from build123d import *

# Parameters (mm, degrees)
SKETCH1_W                       = 12.7
SKETCH1_H                       = 6.35
BOSS_EXTRUDE1_DEPTH             = 105.41
SKETCH2_W                       = 12.7
SKETCH2_H                       = 6.35
BOSS_EXTRUDE2_DEPTH             = 127
SKETCH3_W                       = 12.7
SKETCH3_H                       = 6.35
BOSS_EXTRUDE3_DEPTH             = 105.41
CUT_EXTRUDE1_DEPTH              = 128
LPATTERN1_COUNT                 = 5
LPATTERN1_PITCH                 = 19.05
F_9_64_0_14063_DIAMETER_HOLE1_D = 3.572002


with BuildPart() as part:
    # Sketch1 → Boss-Extrude1 (new body)
    with BuildSketch(Plane(origin=(0, 0, 0), x_dir=(1, 0, 0), z_dir=(0, 1, 0))):
        Rectangle(SKETCH1_W, SKETCH1_H)
    extrude(amount=-BOSS_EXTRUDE1_DEPTH)

    # Sketch2 → Boss-Extrude2 (add)
    with BuildSketch(Plane.XY.offset(3.175)):
        with Locations((0, -102.235)):
            Rectangle(SKETCH2_W, SKETCH2_H)
    extrude(amount=-BOSS_EXTRUDE2_DEPTH)

    # Sketch3 → Boss-Extrude3 (add)
    with BuildSketch(Plane.XZ.offset(105.41)):
        with Locations((0, -120.65)):
            Rectangle(SKETCH3_W, SKETCH3_H)
    extrude(amount=-BOSS_EXTRUDE3_DEPTH)

    # Sketch4 → Cut-Extrude1 (cut, through all)
    with BuildSketch(Plane(origin=(0, 0, -123.825), x_dir=(-1, 0, 0), z_dir=(0, 0, -1))):
        with BuildLine():
            Line((3.175, -10.16), (3.175, -17.78))
            ThreePointArc((3.175, -17.78), (0, -20.955), (-3.175, -17.78))
            Line((-3.175, -17.78), (-3.175, -10.16))
            ThreePointArc((-3.175, -10.16), (0, -6.985), (3.175, -10.16))
        make_face()
    cut_extrude1 = extrude(amount=-CUT_EXTRUDE1_DEPTH, mode=Mode.SUBTRACT)

    # LPattern1: Cut-Extrude1 ×5
    with Locations(*[(0, -i * LPATTERN1_PITCH, 0) for i in range(1, LPATTERN1_COUNT)]):
        add(cut_extrude1, mode=Mode.SUBTRACT)

    # 9/64 (0.14063) Diameter Hole1 (through all)
    with Locations(Plane(origin=(0, 0, -123.825), x_dir=(-1, 0, 0), z_dir=(0, 0, -1))):
        with Locations((0, -2.667)):
            Hole(F_9_64_0_14063_DIAMETER_HOLE1_D / 2)


solid = part.part
Geometry check sheet. Reference: the model listing, model coordinates, mm. A direction names the side the tool comes from. Give positions to 0.01 mm unless a question says otherwise; leave off trailing zeros. Write each loop counter-clockwise with the first axis right and the second up, starting at its lowest first coordinate (ties: lowest second). Pieces come first, ordered by that corner, then holes. Notation, with made-up numbers: M -26.5,-15 L -2.5,-15 A20 cw -2.5,10 Z; hole C -20,43.25 d10. An arc over 180 degrees is marked long. Answer as CSV lines item,"result". Start each with the question number.
Q1. Section check B-B, the plane x = -5. Record the cut outline in (y, z) (3 decimals).
Q2. Release check for a two-part mould opening along X. For faces 1 (the face through (3.175, -90, 0)), 2 (the face through (0, -99.06, -60)) record: pulls with the +X half, pulls with the -X half, needs draft (parallel to the pull), parting line crosses it, or undercut.
Q3. Section check D-D, the plane y = -8.5. Record the cut outline in (x, z) (3 decimals).
Q4. Section check C-C, the plane z = -12.5. Record the cut outline in (x, y), then the cut area to 3 significant figures.
Q5. Section check A-A, the plane y = -71. Record the cut outline in (x, z) (3 decimals), then the cut area to 3 significant figures.
Q6. Tool access check on faces 3 (the face through (-0.07, -97.154, -120.694)), 4 (the face through (0, 0, 0)). Record the directions out of +Z, -Z, +X, -X, +Y, -Y that give a thin tool (end or side, any length) a straight path to the whole face; none if there is none.
Q7. Go/stop test with a flat-tipped pin: pin 1 (3 mm diameter, centred on x = -3, z = -89, fed in from +Y). Record where the tip stops, or that it passes through.
Q8. Material ranges on L1, parallel to Z at x = 5.5, y = -92 (3 decimals); L2, parallel to X at y = -88.5, z = -3 (3 decimals); L3, parallel to Y at x = -5, z = -91.5, recorded low to high.
Geometry says:
1,outline,"M -105.41,-123.825 L 0,-123.825 L 0,-117.475 L -99.06,-117.475 L -99.06,-3.175 L 0,-3.175 L 0,3.175 L -105.41,3.175 Z"
2,face 1,"undercut"
2,face 2,"needs draft"
3,outline,"M -6.35,-123.825 L -2.706,-123.825 L -2.706,-117.475 L -6.35,-117.475 Z; M -6.35,-3.175 L -2.706,-3.175 L -2.706,3.175 L -6.35,3.175 Z; M 2.706,-123.825 L 6.35,-123.825 L 6.35,-117.475 L 2.706,-117.475 Z; M 2.706,-3.175 L 6.35,-3.175 L 6.35,3.175 L 2.706,3.175 Z"
4,outline,"M -6.35,-105.41 L 6.35,-105.41 L 6.35,-99.06 L -6.35,-99.06 Z"
4,area,"80.6 mm^2"
5,outline,"M -6.35,-123.825 L -3.175,-123.825 L -3.175,-117.475 L -6.35,-117.475 Z; M -6.35,-3.175 L -3.175,-3.175 L -3.175,3.175 L -6.35,3.175 Z; M 3.175,-123.825 L 6.35,-123.825 L 6.35,-117.475 L 3.175,-117.475 Z; M 3.175,-3.175 L 6.35,-3.175 L 6.35,3.175 L 3.175,3.175 Z"
5,area,"80.6 mm^2"
6,face 3,"+Z, -Z"
6,face 4,"+Z, -Z, +X, -X, +Y"
7,pin 1,"y = -99.06"
8,L1,"-123.825 to -117.475, -3.175 to 3.175"
8,L2,"-6.35 to -3.175, 3.175 to 6.35"
8,L3,"-105.41 to -99.06"
